Could you check a few things on this model? Use its own coordinates, in mm. Face numbers are marked on the shaded views. Round coordinates to 2 decimals unless told otherwise and drop trailing zeros. Write each loop counter-clockwise with the first axis right and the second up, starting at its lowest first coordinate (ties: lowest second). Pieces come first, ordered by that corner, then holes. Notation, with made-up numbers: (-31, -32.75) -> (24, -32.75) arc R14 ccw to (24, -5.75) -> close; hole circle Ø9 at (81.5, -3). An arc over 180 degrees is marked (long way). Answer as CSV lines item,"result". Start each with the question number.
Q1. Imagine slicing it at C-C on x = -42. Please give me the cut outline in (y, z), and give its area (3 significant figures).
Q2. If we mould it in two halves opening along Y, with no side actions, what happens to the marked faces 1, 2 and 3? For each: pulls with the +Y half, pulls with the -Y half, needs draft (parallel to the pull), parting line crosses it, or undercut.
Q3. Imagine slicing it at A-A on z = -35. Please give me the cut outline in (x, y).
Q4. Will these pins go through, and if not, where does the flat tip stop? pin 1 Ø8 at (y, z) = (82.5, 7.5) entering from -X; pin 2 Ø6 at (y, z) = (-14, -19) entering from -X; pin 3 Ø3 at (x, y) = (-12, 70.5) entering from +Z.
Q5. Imagine slicing it at B-B on y = 45. Please give me the cut outline in (x, z).
Q6. If I drill on line 1 (Z direction, x = -26, y = 56.5); line 2 (Z direction, x = 13, y = 26); line 3 (X direction, y = 74.5, z = 12.5), over which ranges is the centre line in solid material (lowest first)? Write a range as [from, to].
from build123d import *

# Parameters (mm, degrees)
BOSS_EXTRUDE1_DEPTH = 69.85
SKETCH3_R           = 11.43
SKETCH3_R_2         = 8.89
CUT_EXTRUDE1_DEPTH  = 0.635
SKETCH3_4_R         = 8.89
SKETCH3_4_R_2       = 7.62
CUT_EXTRUDE2_DEPTH  = 5.08
SKETCH3_5_R         = 7.62
CUT_EXTRUDE3_DEPTH  = 0.508
FILLET1_R           = 2.54
SKETCH3_6_R         = 15.24
SKETCH3_6_R_2       = 6.35
CUT_EXTRUDE4_DEPTH  = 0.635
SKETCH3_7_R         = 6.35
CUT_EXTRUDE5_DEPTH  = 6.35
FILLET5_R           = 6.35
SKETCH7_R           = 0.764119483
BOSS_EXTRUDE3_DEPTH = 0.254
SKETCH7_4_R         = 0.635
CUT_EXTRUDE6_DEPTH  = 0.127
SKETCH8_R           = 3.175
CUT_EXTRUDE7_DEPTH  = 2.54
SCALE1_SCALE        = 2


with BuildPart() as part:
    # Sketch1 → Boss-Extrude1 (new body)
    with BuildSketch(Plane(origin=(0, 0, 0), x_dir=(1, 0, 0), z_dir=(0, 1, 0))):
        Polygon((-25.4, 0), (25.4, 0), (15.538994382, 36.801773982), (-15.538994382, 36.801773982), align=None)
    extrude(amount=BOSS_EXTRUDE1_DEPTH)

    # Sketch3 → Cut-Extrude1 (cut)
    with BuildSketch(Plane.XY):
        with Locations((0, 53.34)):
            Circle(SKETCH3_R)
        with Locations((0, 53.34)):
            Circle(SKETCH3_R_2, mode=Mode.SUBTRACT)
    extrude(amount=-CUT_EXTRUDE1_DEPTH, mode=Mode.SUBTRACT)

    # Sketch3<4> → Cut-Extrude2 (cut)
    with BuildSketch(Plane.XY):
        with Locations((0, 53.34)):
            Circle(SKETCH3_4_R)
        with Locations((0, 53.34)):
            Circle(SKETCH3_4_R_2, mode=Mode.SUBTRACT)
    extrude(amount=-CUT_EXTRUDE2_DEPTH, mode=Mode.SUBTRACT)

    # Sketch3<5> → Cut-Extrude3 (cut)
    with BuildSketch(Plane.XY):
        with Locations((0, 53.34)):
            Circle(SKETCH3_5_R)
    extrude(amount=-CUT_EXTRUDE3_DEPTH, mode=Mode.SUBTRACT)

    # Fillet1
    fillet1_edges = [part.edges().sort_by_distance(p)[0] for p in [
        (-7.62, 53.34, -0.508),
    ]]
    fillet(fillet1_edges, radius=FILLET1_R)

    # Sketch3<6> → Cut-Extrude4 (cut)
    with BuildSketch(Plane.XY):
        with Locations((0, 19.05)):
            Circle(SKETCH3_6_R)
        with Locations((0, 19.05)):
            Circle(SKETCH3_6_R_2, mode=Mode.SUBTRACT)
    extrude(amount=-CUT_EXTRUDE4_DEPTH, mode=Mode.SUBTRACT)

    # Sketch3<7> → Cut-Extrude5 (cut)
    with BuildSketch(Plane.XY):
        with Locations((0, 19.05)):
            Circle(SKETCH3_7_R)
    extrude(amount=-CUT_EXTRUDE5_DEPTH, mode=Mode.SUBTRACT)

    # Fillet5
    # the kernel refuses this fillet: 6.35 mm, written as the material it takes off along each edge
    with BuildSketch(Plane(origin=(0, 19.05, -0.635), x_dir=(1, 0, 0), z_dir=(0, -1, 0))) as fillet5_piece_1:
        with BuildLine():
            CenterArc((12.668170226, -6.35), FILLET5_R, 90, 84.260829523)
            Line((6.35, -5.715), (6.223636595, -5.7023))
            ThreePointArc((6.223636595, -5.7023), (6.223, -2.8575), (6.223, 0))
            Line((6.223, 0), (6.35, 0.127))
            Line((6.35, 0.127), (12.668170226, 0.127))
            Line((12.668170226, 0.127), (12.668170226, 0))
        make_face()
    revolve(axis=Axis((0, 19.05, -0.635), (0, 0, 1)), mode=Mode.SUBTRACT)

    # Sketch7 → Boss-Extrude3 (add)
    with BuildSketch(Plane.XY):
        with Locations(Location((21.59, 3.81, 0), (0, 0, 180))):
            Circle(SKETCH7_R)
    extrude(amount=BOSS_EXTRUDE3_DEPTH)

    # Sketch7<4> → Cut-Extrude6 (cut)
    with BuildSketch(Plane.XY):
        with Locations((19.05, 3.81)):
            Circle(SKETCH7_4_R)
    extrude(amount=-CUT_EXTRUDE6_DEPTH, mode=Mode.SUBTRACT)

    # Sketch8 → Cut-Extrude7 (cut)
    with BuildSketch(Plane.XZ):
        with Locations(Location((0, -27.94, 0), (0, 0, 270))):
            Circle(SKETCH8_R)
    extrude(amount=-CUT_EXTRUDE7_DEPTH, mode=Mode.SUBTRACT)


with BuildPart() as part_1:
    # Scale1: scaled about (6.7929e-05, 35.092141807, -17.231977993)
    add(part.part.scale(SCALE1_SCALE).moved(Location((-6.7929e-05, -35.092141807, 17.231977993))))


solid = part_1.part
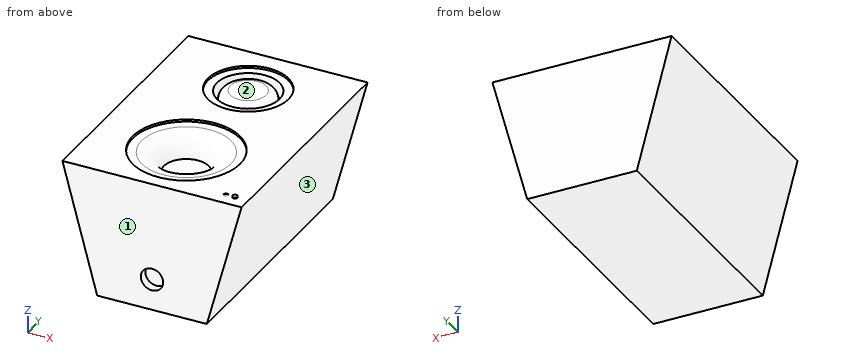
Checks:
1,outline,"(-35.09, -15.61) -> (104.61, -15.61) -> (104.61, 17.23) -> (-35.09, 17.23) -> close"
1,area,"4,590 mm^2"
2,face 1,"pulls with the -Y half"
2,face 2,"undercut"
2,face 3,"needs draft"
3,outline,"(-36.8, -35.09) -> (-5.2, -35.09) -> (-5.2, -30.01) -> (5.2, -30.01) -> (5.2, -35.09) -> (36.8, -35.09) -> (36.8, 104.61) -> (-36.8, 104.61) -> close"
4,pin 1,"x = -49.26"
4,pin 2,"x = -41.9"
4,pin 3,"z = 16.2"
5,outline,"(-50.8, 17.23) -> (-31.08, -56.37) -> (31.08, -56.37) -> (50.8, 17.23) -> close"
6,line 1,"[-56.37, 17.23]"
6,line 2,"[-56.37, 15.96]"
6,line 3,"[-49.53, -17.54], [-14.77, 14.77], [17.54, 49.53]"
